Part model, mm, in its own coordinate system. Round coordinates to 2 decimals unless told otherwise and drop trailing zeros. Write each loop counter-clockwise with the first axis right and the second up, starting at its lowest first coordinate (ties: lowest second). Pieces come first, ordered by that corner, then holes. Notation, with made-up numbers: M 17,-14 L 58,-14 A16 cw 58,-3 Z; hole C 20.25,-39 d11. An arc over 180 degrees is marked long. One line per question, with ' | ' between items. Start each with the question number.
1) Saw through at A-A (z = -67). List the corners of the cut face in (x, y), plus the area to 3 significant figures.
2) Saw through at B-B (x = -15). List the corners of the cut face in (y, z).
3) Wall check: probe 1 along X at (y, z) = (-5, -67); probe 2 along Z at (x, y) = (14, 2). Give the ranges that are in metal, low to high. Write a range as [from, to].
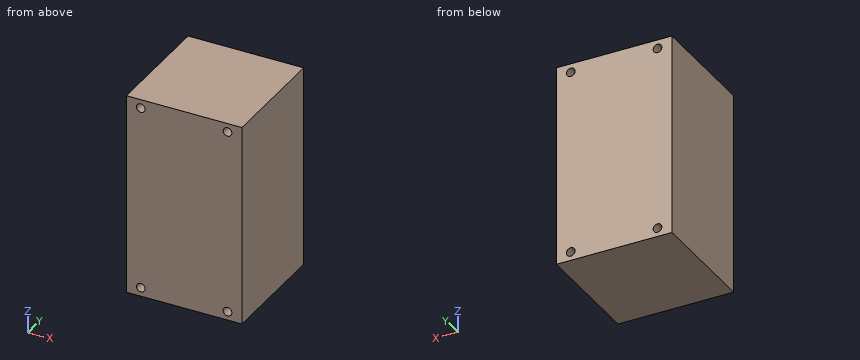
```python
from build123d import *

# Parameters (mm, degrees)
SKETCH_1_W            = 40
SKETCH_1_H            = 40
EXTRUDE_1_DEPTH       = 70
HOLE_WIZARD_3_0_3_1_D = 3


with BuildPart() as part:
    # 草图1 → 凸台-拉伸1 (new body)
    with BuildSketch(Plane.XY):
        Rectangle(SKETCH_1_W, SKETCH_1_H)
    extrude(amount=-EXTRUDE_1_DEPTH)

    # Ø3.0 (3) 直径孔1 (through all)
    with Locations(Plane(origin=(-15, 20, -67), x_dir=(0, 0, 1), z_dir=(0, 1, 0))):
        with Locations((0, 0), (0, 30), (64, 0), (64, 30)):
            Hole(HOLE_WIZARD_3_0_3_1_D / 2)


solid = part.part
```
Answer key:
1) outline: M -20,-20 L -16.5,-20 L -16.5,20 L -20,20 Z; M -13.5,-20 L 13.5,-20 L 13.5,20 L -13.5,20 Z; M 16.5,-20 L 20,-20 L 20,20 L 16.5,20 Z | area: 1,360 mm2
2) outline: M -20,-70 L 20,-70 L 20,-68.5 L -20,-68.5 Z; M -20,-65.5 L 20,-65.5 L 20,-4.5 L -20,-4.5 Z; M -20,-1.5 L 20,-1.5 L 20,0 L -20,0 Z
3) probe 1: x = [-20, -16.5], [-13.5, 13.5], [16.5, 20] | probe 2: z = [-70, -68.12], [-65.88, -4.12], [-1.88, 0]
